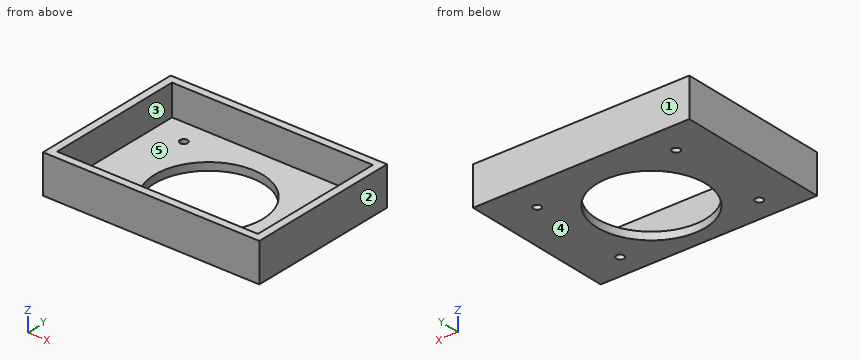
from build123d import *

# Parameters (mm, degrees)
F0_W     = 140
F0_H     = 100
F0_W_2   = 130
F0_H_2   = 90
F1_DEPTH = 25
F0_R     = 2.5
F0_R_2   = 35
F2_DEPTH = 5


with BuildPart() as f1:
    # F0 (on Top) → F1 (new body)
    with BuildSketch(Plane.XY):
        with Locations((70, 50)):
            Rectangle(F0_W, F0_H)
        with Locations((70, 50)):
            Rectangle(F0_W_2, F0_H_2, mode=Mode.SUBTRACT)
    extrude(amount=F1_DEPTH)

    # F0 (on Top) → F2 (join)
    with BuildSketch(Plane.XY):
        with Locations((70, 50)):
            Rectangle(F0_W_2, F0_H_2)
        with Locations((25, 15)):
            Circle(F0_R, mode=Mode.SUBTRACT)
        with Locations((115, 15)):
            Circle(F0_R, mode=Mode.SUBTRACT)
        with Locations((70, 45)):
            Circle(F0_R_2, mode=Mode.SUBTRACT)
        with Locations((25, 80)):
            Circle(F0_R, mode=Mode.SUBTRACT)
        with Locations((115, 80)):
            Circle(F0_R, mode=Mode.SUBTRACT)
    extrude(amount=F2_DEPTH)


solid = f1.part
Work out the finished part from the listing and answer in its coordinate system (mm). Face numbers are marked on the shaded views. A direction names the side the tool comes from. Give positions to 0.01 mm unless a question says otherwise; leave off trailing zeros. Order: outer loops, then holes, each group sorted by start corner. A loop starts at its lowest first (then second) coordinate and runs counter-clockwise, first axis right, second up. Notation, with made-up numbers: M -13,4 L 4,4 A27 cw 4,41 Z; hole C 44,-13.75 d11. An arc over 180 degrees is marked long. Return JSON: item names as keys, results as strings.
Q1. This flat-tipped pin is pushed along its axis until it touches: pin 1 (6.5 mm diameter, centred on x = 115, y = 80, fed in from +Z). Where does it stop, or does it pass through?
Answer below:
{"pin 1": "stops at z = 5"}
Q2. Find section C-C, the plane z = 21.5. Write down the section's boundary in (x, y).
Answer below:
{"outline": "M 0,0 L 140,0 L 140,100 L 0,100 Z; hole M 5,5 L 135,5 L 135,95 L 5,95 Z"}
Q3. Find section D-D, the plane x = 115. Write down the section's boundary in (y, z).
Answer below:
{"outline": "M 0,0 L 12.5,0 L 12.5,5 L 5,5 L 5,25 L 0,25 Z; M 17.5,0 L 77.5,0 L 77.5,5 L 17.5,5 Z; M 82.5,0 L 100,0 L 100,25 L 95,25 L 95,5 L 82.5,5 Z"}
Q4. The mould has two halves that part along Y. Classify the marked faces 1, 2 and 3: pulls with the +Y half, pulls with the -Y half, needs draft (parallel to the pull), parting line crosses it, or undercut.
Answer below:
{"face 1": "pulls with the +Y half", "face 2": "needs draft", "face 3": "undercut"}
Q5. Which of the six approach directions +Z, -Z, +X, -X, +Y, -Y give full straight-line access (tool end or side, diameter ignored) to the marked faces 4 and 5?
Answer below:
{"face 4": "-Z, +X, -X, +Y, -Y", "face 5": "+Z"}
Q6. Find section B-B, the plane x = 70. Write down the section's boundary in (y, z), and give its area (3 significant figures).
Answer below:
{"outline": "M 0,0 L 10,0 L 10,5 L 5,5 L 5,25 L 0,25 Z; M 80,0 L 100,0 L 100,25 L 95,25 L 95,5 L 80,5 Z", "area": "350 mm^2"}
Q7. Find section A-A, the plane y = 45. Write down the section's boundary in (x, z), and give its area (3 significant figures).
Answer below:
{"outline": "M 0,0 L 35,0 L 35,5 L 5,5 L 5,25 L 0,25 Z; M 105,0 L 140,0 L 140,25 L 135,25 L 135,5 L 105,5 Z", "area": "550 mm^2"}
Q8. Find the intervals of material crossed by line 1 along Y through (x, z) = (115, 1.95); line 2 along Y through (x, z) = (58.5, 19.75); line 3 along X through (y, z) = (11.5, 19), in increasing order. Write a range as [from, to].
Answer below:
{"line 1": "y = [0, 12.5], [17.5, 77.5], [82.5, 100]", "line 2": "y = [0, 5], [95, 100]", "line 3": "x = [0, 5], [135, 140]"}
